Could you check a few things on this model? Use its own coordinates, in mm. Give positions to 0.01 mm unless a question says otherwise; leave off trailing zeros. Loops run counter-clockwise (first coordinate to the right, second up) from the corner with the lowest first, then second, coordinate; pieces in that order, holes last. Notation, with made-up numbers: M 32.25,30 L 50.25,30 A22 cw 50.25,56 Z; hole C 9.5,26 d4. An arc over 180 degrees is marked long. Answer in a Markdown table with one row per item. Add a question column.
1. If we section it at D-D on y = 215.5: List the corners of the cut face in (x, z) for me.
2. I'm going to push flat-ended pins straight in: pin 1 Ø1.9 at (x, z) = (4, 103.5) entering from +Y; pin 2 Ø1 at (x, y) = (2, 169.5) entering from -Z; pin 3 Ø1.9 at (x, y) = (3.5, 294.5) entering from -Z; pin 4 Ø2 at (y, z) = (278.74, -360.04) entering from -X. Where does each tip first touch, or does it pass through?
3. Thinking about a two-plate mould opening in Z: for faces 1 (the flat face through (6.35, 149, -118)), 2 (the flat face through (3.22, 285.82, -446.55)), 3 (the flat face through (3.131, 303.901, -471.865)), which applies, released by +Z, released by -Z, zero draft, split by the parting line, or undercut?
4. If we section it at C-C on y = 302: List the corners of the cut face in (x, z) for me.
5. If we section it at B-B on x = 3.25: Count the separate pieces of the cut face and the enclosed holes in it, then the cut area to 3 significant figures.
6. If we section it at A-A on y = 27.5: List the corners of the cut face in (x, z) for me.
7. I need wall thicknesses on line 1 along Z through (x, y) = (4.5, 234.5); line 2 along Z through (x, y) = (4.5, 74); line 3 along Z through (x, y) = (5.25, 231). Which ranges of each line are inside material? Lowest first, please. Write a range as from..to.
```python
from build123d import *

# Parameters (mm, degrees)
BOSS_EXTRUDE1_DEPTH                            = 6.35
SKETCH2_W                                      = 25.4
SKETCH2_H                                      = 304.8
CUT_EXTRUDE1_DEPTH                             = 589.439392722
CUT_EXTRUDE2_DEPTH                             = 589.439392722
CSK_FOR_4_FLAT_HEAD_MACHINE_SCREW3_D           = 3.2639
CSK_FOR_4_FLAT_HEAD_MACHINE_SCREW3_CSINK_D     = 5.715
CSK_FOR_4_FLAT_HEAD_MACHINE_SCREW3_CSINK_ANGLE = 82
CSK_FOR_4_FLAT_HEAD_MACHINE_SCREW2_D           = 3.2639
CSK_FOR_4_FLAT_HEAD_MACHINE_SCREW2_CSINK_D     = 5.715
CSK_FOR_4_FLAT_HEAD_MACHINE_SCREW2_CSINK_ANGLE = 82
CSK_FOR_4_FLAT_HEAD_MACHINE_SCREW1_D           = 3.2639
CSK_FOR_4_FLAT_HEAD_MACHINE_SCREW1_CSINK_D     = 5.715
CSK_FOR_4_FLAT_HEAD_MACHINE_SCREW1_CSINK_ANGLE = 82
CSK_FOR_4_FLAT_HEAD_MACHINE_SCREW4_D           = 3.2639
CSK_FOR_4_FLAT_HEAD_MACHINE_SCREW4_CSINK_D     = 5.715
CSK_FOR_4_FLAT_HEAD_MACHINE_SCREW4_CSINK_ANGLE = 82
CHAMFER1_SIZE                                  = 10.558581723
CHAMFER1_SIZE_2                                = 6.096
CUT_EXTRUDE3_REACH                             = 587.916
SKETCH7_W                                      = 25.4
SKETCH7_H                                      = 49.005174209


with BuildPart() as part:
    # Sketch1 → Boss-Extrude1 (new body)
    with BuildSketch(Plane(origin=(0, 0, 0), x_dir=(0, 0, -1), z_dir=(1, 0, 0))):
        Polygon((487.035764647, 330.176862244), (276.230747609, -34.948137756), (-122.564235353, -34.948137756), (-122.564235353, 330.176862244), align=None)
    extrude(amount=BOSS_EXTRUDE1_DEPTH)

    # Sketch2 → Cut-Extrude1 (cut, through all)
    with BuildSketch(Plane(origin=(6.35, 0, 0), x_dir=(0, 0, -1), z_dir=(1, 0, 0))):
        with Locations((245.735764647, 168.251862244)):
            Rectangle(SKETCH2_W, SKETCH2_H)
    extrude(amount=-CUT_EXTRUDE1_DEPTH, mode=Mode.SUBTRACT)

    # Sketch3 → Cut-Extrude2 (cut, through all)
    with BuildSketch(Plane(origin=(6.35, 0, 0), x_dir=(0, 0, -1), z_dir=(1, 0, 0))):
        Polygon((457.706370973, 279.376862244), (276.230747609, -34.948137756), (246.901353935, -34.948137756), (435.709325716, 292.076862244), align=None)
    extrude(amount=-CUT_EXTRUDE2_DEPTH, mode=Mode.SUBTRACT)

    # CSK for #4 Flat Head Machine Screw3 (through all)
    with Locations(Plane(origin=(6.35, 253.341862244, 109.864235353), x_dir=(0, 0, 1), z_dir=(1, 0, 0))):
        with Locations((0, 0), (-317.5, 0), (-469.9, -25.4)):
            CounterSinkHole(CSK_FOR_4_FLAT_HEAD_MACHINE_SCREW3_D / 2, CSK_FOR_4_FLAT_HEAD_MACHINE_SCREW3_CSINK_D / 2, counter_sink_angle=CSK_FOR_4_FLAT_HEAD_MACHINE_SCREW3_CSINK_ANGLE)

    # CSK for #4 Flat Head Machine Screw2 (through all)
    with Locations(Plane(origin=(6.35, 100.941862244, 109.864235353), x_dir=(0, 0, 1), z_dir=(1, 0, 0))):
        with Locations((0, 0)):
            CounterSinkHole(CSK_FOR_4_FLAT_HEAD_MACHINE_SCREW2_D / 2, CSK_FOR_4_FLAT_HEAD_MACHINE_SCREW2_CSINK_D / 2, counter_sink_angle=CSK_FOR_4_FLAT_HEAD_MACHINE_SCREW2_CSINK_ANGLE)

    # CSK for #4 Flat Head Machine Screw1 (through all)
    with Locations(Plane(origin=(6.35, -9.548137756, 46.364235353), x_dir=(0, 0, 1), z_dir=(1, 0, 0))):
        with Locations((0, 0), (-254, 0)):
            CounterSinkHole(CSK_FOR_4_FLAT_HEAD_MACHINE_SCREW1_D / 2, CSK_FOR_4_FLAT_HEAD_MACHINE_SCREW1_CSINK_D / 2, counter_sink_angle=CSK_FOR_4_FLAT_HEAD_MACHINE_SCREW1_CSINK_ANGLE)

    # CSK for #4 Flat Head Machine Screw4 (through all)
    with Locations(Plane(origin=(6.35, 235.418036453, -355.337072673), x_dir=(0, 0, 1), z_dir=(1, 0, 0))):
        with Locations((0, 0), (-31.648510504, -4.016828178), (58.65878735, 101.6), (27.010276846, 97.583171822)):
            CounterSinkHole(CSK_FOR_4_FLAT_HEAD_MACHINE_SCREW4_D / 2, CSK_FOR_4_FLAT_HEAD_MACHINE_SCREW4_CSINK_D / 2, counter_sink_angle=CSK_FOR_4_FLAT_HEAD_MACHINE_SCREW4_CSINK_ANGLE)

    # Chamfer1
    # the kernel refuses this chamfer: 10.558581723, 6.096 mm, written as the material it takes off along each edge
    with BuildSketch(Plane(origin=(0, 330.176862244, 149.880191717), x_dir=(0.9998132206222078, 0.01932676561270281, 0), z_dir=(0, 0, -1))) as chamfer1_piece_1:
        Polygon((CHAMFER1_SIZE * 0.999813220617, CHAMFER1_SIZE * 0.0193267656126), (-CHAMFER1_SIZE_2 * 0.0193267656127, CHAMFER1_SIZE_2 * 0.999813220622), (0, 0), align=None)
    extrude(amount=664.231912729, mode=Mode.SUBTRACT)

    # Sketch7 → Cut-Extrude3 (cut, up to next)
    with BuildSketch(Plane(origin=(6.35, 0, 0), x_dir=(0, 0, -1), z_dir=(1, 0, 0)), mode=Mode.PRIVATE) as cut_extrude3_sk1:
        with Locations((-100.339235353, 303.244449348)):
            Rectangle(SKETCH7_W, SKETCH7_H)
    cut_extrude3_tool1 = extrude(cut_extrude3_sk1.sketch, amount=-CUT_EXTRUDE3_REACH, mode=Mode.PRIVATE) & part.part
    add(cut_extrude3_tool1.solids().sort_by_distance((6.35, 303.244449, 100.339235))[0], mode=Mode.SUBTRACT)


solid = part.part
```
Results:
| question | item | result |
|---|---|---|
| 1 | outline | M 0,-391.5 L 6.35,-391.5 L 6.35,-258.44 L 0,-258.44 Z; M 0,-233.04 L 6.35,-233.04 L 6.35,122.56 L 0,122.56 Z |
| 2 | pin 1 | y = 278.74 |
| 2 | pin 2 | z = -365.23 |
| 2 | pin 3 | z = -466.99 |
| 2 | pin 4 | through |
| 3 | face 1 | zero draft |
| 3 | face 2 | undercut |
| 3 | face 3 | released by -Z |
| 4 | outline | M 0,-470.77 L 6.35,-470.77 L 6.35,-258.44 L 0,-258.44 Z; M 0,-233.04 L 6.35,-233.04 L 6.35,87.64 L 0,87.64 Z; M 0,113.04 L 6.35,113.04 L 6.35,122.56 L 0,122.56 Z |
| 5 | separate pieces | 1 |
| 5 | enclosed holes | 11 |
| 5 | area | 163,000 mm2 |
| 6 | outline | M 0,-282.96 L 6.35,-282.96 L 6.35,-258.44 L 0,-258.44 Z; M 0,-233.04 L 6.35,-233.04 L 6.35,122.56 L 0,122.56 Z |
| 7 | line 1 | -402.47..-356.69, -353.99..-258.44, -233.04..122.56 |
| 7 | line 2 | -309.8..-258.44, -233.04..122.56 |
| 7 | line 3 | -400.45..-258.44, -233.04..122.56 |
